Part model, mm, in its own coordinate system. Face numbers are marked on the shaded views. A direction names the side the tool comes from. Round coordinates to 2 decimals unless told otherwise and drop trailing zeros. Loops run counter-clockwise (first coordinate to the right, second up) from the corner with the lowest first, then second, coordinate; pieces in that order, holes last.
from build123d import *

# Parameters (mm, degrees)
SKETCH1_W                = 80
SKETCH1_H                = 15
BOSS_EXTRUDE1_DEPTH      = 10
FILLET1_R                = 7.5
BOSS_EXTRUDE2_DEPTH      = 2
BOSS_EXTRUDE2_DEPTH_BACK = 13
SKETCH2_R                = 3.5
SKETCH2_R_2              = 2.5
SKETCH4_W                = 12.275600057
SKETCH4_H                = 15
CUT_EXTRUDE1_DEPTH       = 39
SKETCH6_W                = 10
SKETCH6_H                = 14.887271561
CUT_EXTRUDE2_DEPTH       = 39
SKETCH8_W                = 33
SKETCH8_H                = 28
BOSS_EXTRUDE3_DEPTH      = 15
CUT_EXTRUDE3_DEPTH       = 12
SKETCH10_W               = 33
SKETCH10_H               = 18
CUT_EXTRUDE4_DEPTH       = 2
SKETCH11_W               = 11.438718319
SKETCH11_H               = 15
CUT_EXTRUDE5_DEPTH       = 84.360662185
SKETCH12_R               = 2.5
CUT_EXTRUDE6_DEPTH       = 86.755466298


with BuildPart() as part:
    # Sketch1 → Boss-Extrude1 (new body)
    with BuildSketch(Plane.XY):
        with Locations((40, 7.5)):
            Rectangle(SKETCH1_W, SKETCH1_H)
    extrude(amount=BOSS_EXTRUDE1_DEPTH)

    # Fillet1
    fillet1_edges = [part.edges().sort_by_distance(p)[0] for p in [
        (0, 0, 5),
        (0, 15, 5),
    ]]
    fillet(fillet1_edges, radius=FILLET1_R - 0.0001)  # a hair under: the kernel refuses the full size

    # Sketch2 → Boss-Extrude2 (add, two sides: drawn at the far end of the back side and taken through both)
    # profile 1 of 2: a face of its own
    with BuildSketch(Plane.XY.offset(10).offset(-BOSS_EXTRUDE2_DEPTH_BACK)):
        with Locations((7.5, 7.5)):
            Circle(SKETCH2_R)
        with Locations((7.5, 7.5)):
            Circle(SKETCH2_R_2, mode=Mode.SUBTRACT)
    # profile 2 of 2: a face of its own
    with BuildSketch(Plane.XY.offset(10).offset(-BOSS_EXTRUDE2_DEPTH_BACK)):
        with Locations((72.5, 7.5)):
            Circle(SKETCH2_R)
        with Locations((72.5, 7.5)):
            Circle(SKETCH2_R_2, mode=Mode.SUBTRACT)
    extrude(amount=BOSS_EXTRUDE2_DEPTH + BOSS_EXTRUDE2_DEPTH_BACK)

    # Sketch4 → Cut-Extrude1 (cut)
    with BuildSketch(Plane(origin=(80, 0, 0), x_dir=(0, 0, -1), z_dir=(1, 0, 0))):
        with Locations((6.137800029, 7.5)):
            Rectangle(SKETCH4_W, SKETCH4_H)
    extrude(amount=-CUT_EXTRUDE1_DEPTH, mode=Mode.SUBTRACT)

    # Sketch6 → Cut-Extrude2 (cut)
    with BuildSketch(Plane(origin=(0, 0, 0), x_dir=(0, 0, -1), z_dir=(1, 0, 0))):
        with Locations((-15, 7.443635781)):
            Rectangle(SKETCH6_W, SKETCH6_H)
    extrude(amount=CUT_EXTRUDE2_DEPTH, mode=Mode.SUBTRACT)

    # Sketch8 → Boss-Extrude3 (add)
    with BuildSketch(Plane(origin=(0, 15, 0), x_dir=(1, 0, 0), z_dir=(0, 1, 0))):
        with Locations((63.5, 4)):
            Rectangle(SKETCH8_W, SKETCH8_H)
    extrude(amount=-BOSS_EXTRUDE3_DEPTH)

    # Sketch9 → Cut-Extrude3 (cut)
    with BuildSketch(Plane(origin=(0, 15, 0), x_dir=(1, 0, 0), z_dir=(0, 1, 0))):
        Polygon((48, 17), (48, -9), (79, -9), (79, 17), (79, 18), (48, 18), align=None)
    extrude(amount=-CUT_EXTRUDE3_DEPTH, mode=Mode.SUBTRACT)

    # Sketch10 → Cut-Extrude4 (cut)
    with BuildSketch(Plane.XZ):
        with Locations((63.5, -9)):
            Rectangle(SKETCH10_W, SKETCH10_H)
    extrude(amount=-CUT_EXTRUDE4_DEPTH, mode=Mode.SUBTRACT)

    # Sketch11 → Cut-Extrude5 (cut, through all)
    with BuildSketch(Plane(origin=(80, 0, 0), x_dir=(0, 0, -1), z_dir=(1, 0, 0))):
        with Locations((-15.71935916, 7.5)):
            Rectangle(SKETCH11_W, SKETCH11_H)
    extrude(amount=-CUT_EXTRUDE5_DEPTH, mode=Mode.SUBTRACT)

    # Sketch12 → Cut-Extrude6 (cut, through all)
    with BuildSketch(Plane(origin=(0, 0, 9), x_dir=(-1, 0, 0), z_dir=(0, 0, -1))):
        with Locations((-67.5, 9)):
            Circle(SKETCH12_R)
    extrude(amount=-CUT_EXTRUDE6_DEPTH, mode=Mode.SUBTRACT)


solid = part.part
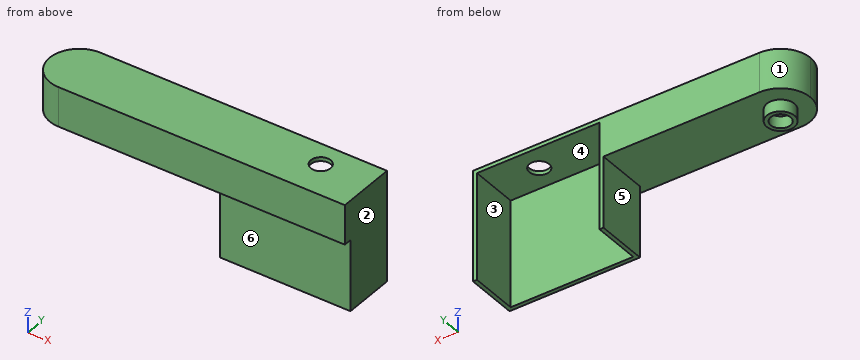
1) Drop flat-ended pins along their axis: pin 1 Ø6 at (x, y) = (64.5, 11.5) entering from -Z; pin 2 Ø3 at (x, z) = (60.5, -3.5) entering from -Y; pin 3 Ø3.5 at (y, z) = (8, -2.5) entering from -X. Give the stop position or say it passes through.
Values:
pin 1: stops at z = 9
pin 2: stops at y = 2
pin 3: stops at x = 4
2) Slice it at C-C, the plane y = 9. Give the cut face in (x, z), then the cut area to 3 significant figures.
Values:
outline: (0.15, 0) - (4.34, 0) - (4.34, -3) - (5.5, -3) - (5.5, 0) - (9.5, 0) - (9.5, -3) - (10.66, -3) - (10.66, 0) - (47, 0) - (47, -18) - (48, -18) - (48, 9) - (65, 9) - (65, 10) - (0.15, 10) - close; (70, 9) - (79, 9) - (79, -18) - (80, -18) - (80, 10) - (70, 10) - close
area: 557 mm2
3) Tool access for the marked faces 4, 5 and 6: list every direction of +Z, -Z, +X, -X, +Y, -Y with a clear straight run to the whole face (end or side of a thin tool).
Values:
face 4: -Z, +Y
face 5: -Z, +Y, -Y
face 6: -Z, +X, -X, -Y
4) Wall check: line 1 along X through (y, z) = (7.5, -0.9); line 2 along X through (y, z) = (9, -7); line 3 along Y through (x, z) = (67.5, 9.5). Give the ranges that are in metal, low to high.
Values:
line 1: x = 4 to 5, 10 to 11, 47 to 48, 79 to 80
line 2: x = 47 to 48, 79 to 80
line 3: y = 0 to 6.5, 11.5 to 15
5) Slice it at A-A, the plane x = 67.5. Give the cut face in (y, z), then the cut area to 3 significant figures.
Values:
outline: (0, 0) - (2, 0) - (2, -18) - (3, -18) - (3, 9) - (6.5, 9) - (6.5, 10) - (0, 10) - close; (11.5, 9) - (15, 9) - (15, 10) - (11.5, 10) - close
area: 55.0 mm2
6) Slice it at D-D, the plane y = 12.5. Give the cut face in (x, z).
Values:
outline: (1.91, 0) - (47, 0) - (47, -18) - (48, -18) - (48, 9) - (79, 9) - (79, -18) - (80, -18) - (80, 10) - (1.91, 10) - close
7) Slice it at B-B, the plane z = -9. Give the cut face in (x, y).
Values:
outline: (47, 2) - (80, 2) - (80, 15) - (79, 15) - (79, 3) - (48, 3) - (48, 15) - (47, 15) - close
8) Mould opens along X. For the marked faces 1, 2 and 3 say: released by +X, released by -X, zero draft, split by the parting line, or undercut.
Values:
face 1: released by -X
face 2: released by +X
face 3: undercut
